Source: CAD feature listing. Evaluate the final solid. Frame: model axes, mm. Give positions to 0.01 mm unless a question says otherwise; leave off trailing zeros. Write each loop counter-clockwise with the first axis right and the second up, starting at its lowest first coordinate (ties: lowest second). Pieces come first, ordered by that corner, then holes. Notation, with made-up numbers: M 58,25.25 L 93,25.25 A23 cw 93,44.25 Z; hole C 55,41 d2. An arc over 180 degrees is marked long. Return JSON: item names as keys, results as strings.
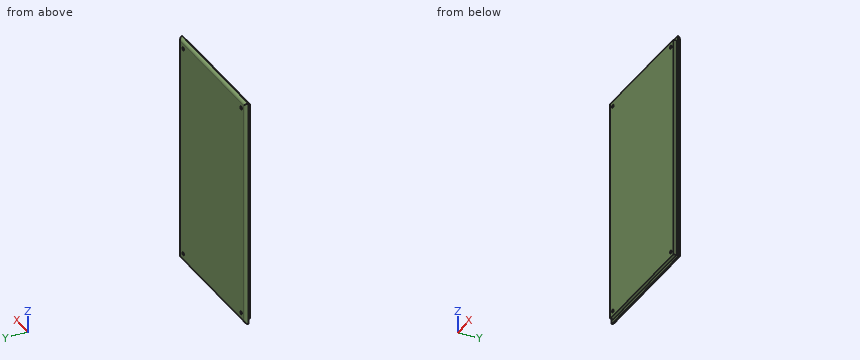
Autodesk Inventor part; units mm, degrees
ref_plane "YZ Plane" through (0, 0, 0) normal (1, 0, 0) x (0, 1, 0)
ref_plane "XZ Plane" through (0, 0, 0) normal (0, 1, 0) x (-1, 0, 0)
ref_plane "XY Plane" through (0, 0, 0) normal (0, 0, 1) x (1, 0, 0)
sketch "Sketch1" plane through (0, 0, 0) normal (0, 1, 0) x (-1, 0, 0)
  line L0 (0, 0) -> (-127.76, 0)
  line L1 (-127.76, 0) -> (-127.76, -226)
  line L2 (-127.76, -226) -> (0, -226)
  line L3 (0, -226) -> (0, 0)
  line L4 (-3, -3) -> (-124.76, -3)
  line L5 (-124.76, -3) -> (-124.76, -223)
  line L6 (-124.76, -223) -> (-3, -223)
  line L7 (-3, -223) -> (-3, -3)
  dimension "d0" = 127.76
  dimension "d1" = 226
  dimension "d2" = 3
extrude "Extrusion1" add sketch "Sketch1" against normal blind 3 contours L7 L6 L5 L4
extrude "Extrusion2" add sketch "Sketch1" along normal blind 3 contours L3 L2 L1 L0 | L7 L6 L5 L4
sketch "Sketch2" plane through (0, 3, 0) normal (0, 1, 0) x (1, 0, 0)
  line L0 (0, 226) -> (0, 0)
  line L1 (0, 113) -> (127.76, 113) construction
  line L2 (127.76, 0) -> (127.76, 226)
  line L3 (0, 0) -> (127.76, 0)
  line L4 (63.88, 0) -> (63.88, 226) construction
  line L5 (127.76, 226) -> (0, 226)
  circle A0 centre (119.76, 8) radius 1.5
  circle A1 centre (8, 8) radius 1.5
  circle A2 centre (119.76, 218) radius 1.5
  circle A3 centre (8, 218) radius 1.5
  dimension "d7" = 3
  dimension "d8" = 8
  dimension "d9" = 8
extrude "Extrusion3" cut sketch "Sketch2" against normal through all contours A0 | A1 | A2 | A3
fillet "Fillet1" radius 3 4 edges at (127.76, 3, -113) (63.88, 3, -226) (0, 3, -113) (63.88, 3, 0)
properties part number "Lid"
1) Cut plane A-A, the plane y = -1.65. Return the cut outline in (x, z).
Numbers:
{"outline": "M 3,-223 L 124.76,-223 L 124.76,-3 L 3,-3 Z; hole C 8,-218 d3; hole C 8,-8 d3; hole C 119.76,-218 d3; hole C 119.76,-8 d3"}
2) Contact query for flat-ended pins moving along their axis: pin 1 Ø1.5 at (x, y) = (94, -1) entering from -Z; pin 2 Ø1.5 at (y, z) = (-2, -73.5) entering from +X; pin 3 Ø3.5 at (x, y) = (52.5, -2) entering from +Z. Output: stop coordinate, or through.
Numbers:
{"pin 1": "stops at z = -223", "pin 2": "stops at x = 124.76", "pin 3": "stops at z = -3"}
3) Line query: line 1 (Z direction, x = 8, y = -1.65); line 2 (X direction, y = -0.85, z = -8); line 3 (X direction, y = 0.5, z = -218). Output: solid intervals per line, ascending. Write a range as [from, to].
Numbers:
{"line 1": "z = [-223, -219.5], [-216.5, -9.5], [-6.5, -3]", "line 2": "x = [3, 6.5], [9.5, 118.26], [121.26, 124.76]", "line 3": "x = [0.04, 6.5], [9.5, 118.26], [121.26, 127.72]"}
